Geometry check sheet. Reference: the model listing, model coordinates, mm. A direction names the side the tool comes from. Coordinates: 2 decimals unless noted, no trailing zeros. Loops run counter-clockwise (first coordinate to the right, second up) from the corner with the lowest first, then second, coordinate; pieces in that order, holes last. Notation, with made-up numbers: (-31.75, 29) -> (-0.75, 29) arc R20 cw to (-0.75, 56) -> close; hole circle Ø10 at (-30, 73.25). An arc over 180 degrees is marked (long way). Answer as a JSON object with one key per item and string values.
from build123d import *

# Parameters (mm, degrees)
SKETCH3_R          = 1.625
CUT_EXTRUDE1_DEPTH = 12
SKETCH4_R          = 2.1
CUT_EXTRUDE2_DEPTH = 10
CHAMFER1_SIZE      = 0.4
CHAMFER2_SIZE      = 0.4
CHAMFER3_SIZE      = 0.4
CHAMFER4_SIZE      = 0.3
CHAMFER5_SIZE      = 0.4


with BuildPart() as part:
    # Sketch2 → Revolve1 (revolve)
    with BuildSketch(Plane(origin=(0, 0, 0), x_dir=(1, 0, 0), z_dir=(0, 1, 0))):
        Polygon((0, 0), (0, 12), (-2.7, 12), (-2.7, 20.075), (-19.2, 20.075), (-19.2, 21.075), (-20.7, 21.075), (-20.7, 17.727837292), (-20.7, 14.575), (-20.7, 8.1), (-15.7, 8.1), (-15.7, 6), (-13.7, 6), (-13.7, 0), align=None)
    revolve(axis=Axis((0, 0, 0), (-1, 0, 0)))

    # Sketch3 → Cut-Extrude1 (cut)
    with BuildSketch(Plane.ZY.offset(20.7)):
        with Locations((0, 16)):
            Circle(SKETCH3_R)
        with Locations((13.856406461, 7.904729806)):
            Circle(SKETCH3_R)
        with Locations((13.773900052, -8.142905292)):
            Circle(SKETCH3_R)
        with Locations((-0.165012817, -16.095270194)):
            Circle(SKETCH3_R)
        with Locations((-14.021419278, -8)):
            Circle(SKETCH3_R)
        with Locations((-13.938912869, 8.047635097)):
            Circle(SKETCH3_R)
    extrude(amount=-CUT_EXTRUDE1_DEPTH, mode=Mode.SUBTRACT)

    # Sketch4 → Cut-Extrude2 (cut)
    with BuildSketch(Plane(origin=(-2.7, 0, 0), x_dir=(0, 0, -1), z_dir=(1, 0, 0))):
        with Locations((-8.125, 14.072912811)):
            Circle(SKETCH4_R)
        with Locations((8.125, 14.072912811)):
            Circle(SKETCH4_R)
        with Locations((16.25, 0)):
            Circle(SKETCH4_R)
        with Locations((8.125, -14.072912811)):
            Circle(SKETCH4_R)
        with Locations((-8.125, -14.072912811)):
            Circle(SKETCH4_R)
        with Locations((-16.25, 0)):
            Circle(SKETCH4_R)
    extrude(amount=-CUT_EXTRUDE2_DEPTH, mode=Mode.SUBTRACT)

    # Chamfer1
    chamfer1_edges = [part.edges().sort_by_distance(p)[0] for p in [
        (-2.7, 0, 20.075),
    ]]
    chamfer(chamfer1_edges, length=CHAMFER1_SIZE)

    # Chamfer2
    chamfer2_edges = [part.edges().sort_by_distance(p)[0] for p in [
        (-20.7, 0, 8.1),
    ]]
    chamfer(chamfer2_edges, length=CHAMFER2_SIZE)

    # Chamfer3
    chamfer3_edges = [part.edges().sort_by_distance(p)[0] for p in [
        (-20.7, 16, -1.625),
        (-20.7, 8.047635097, -15.563912869),
        (-20.7, -8, -15.646419278),
        (-20.7, -16.095270194, -1.790012817),
        (-20.7, -8.142905292, 12.148900052),
        (-20.7, 7.904729806, 12.231406461),
    ]]
    chamfer(chamfer3_edges, length=CHAMFER3_SIZE)

    # Chamfer4
    chamfer4_edges = [part.edges().sort_by_distance(p)[0] for p in [
        (-2.7, 0, 18.35),
        (-2.7, -14.072912811, 10.225),
        (-2.7, -14.072912811, -6.025),
        (-2.7, 0, -14.15),
        (-2.7, 14.072912811, -6.025),
        (-2.7, 14.072912811, 10.225),
    ]]
    chamfer(chamfer4_edges, length=CHAMFER4_SIZE)

    # Chamfer5
    chamfer5_edges = [part.edges().sort_by_distance(p)[0] for p in [
        (-20.7, 0, 21.075),
    ]]
    chamfer(chamfer5_edges, length=CHAMFER5_SIZE)


solid = part.part
1. Thickness scan on probe 1 along Z at (x, y) = (-12.5, -1); probe 2 along X at (y, z) = (-16.5, 10); probe 3 along Y at (x, z) = (-5, 0) (3 decimals). Record the ranges inside material, lowest first. Write a range as from..to.
Evaluation:
{"probe 1": "z = -20.05..-18.1, -14.4..14.4, 18.1..20.05", "probe 2": "x = -20.7..-2.7", "probe 3": "y = -20.075..20.075"}
2. Section check B-B, the plane x = -16.25. Record the boundary of the cut face in (y, z) (3 decimals).
Evaluation:
{"outline": "circle Ø40.15 at (0, 0); hole circle Ø3.25 at (-16.095, -0.165); hole circle Ø3.25 at (-8.143, 13.774); hole circle Ø3.25 at (-8, -14.021); hole circle Ø16.2 at (0, 0); hole circle Ø3.25 at (7.905, 13.856); hole circle Ø3.25 at (8.048, -13.939); hole circle Ø3.25 at (16, 0)"}
3. Mould release check, pull along Z, two halves, no side actions. Record for faces 1 (the face through (-19.758, 12.824, 16.724)), 2 (the face through (-15.7, 3, 5.4)): released by +Z, released by -Z, zero draft, split by the parting line, or undercut.
Evaluation:
{"face 1": "split by the parting line", "face 2": "undercut"}
4. Depth check by flat-ended pin: P1, Ø3, axis at x = -12, y = 2, coming from the -Z side; P2, Ø2, axis at x = -10, y = -16.5, coming from the +Z side; P3, Ø10, axis at x = -13.5, z = -16, coming from the +Y side. Enter the tip coordinate at first touch or a pass-through.
Evaluation:
{"P1": "stops at z = -20.07", "P2": "stops at z = 12.76", "P3": "stops at y = 16.79"}
5. Tool access check on faces 3 (the face through (-11.26, -6.03, -19.15)), 4 (the face through (-14.581, 6.916, 12.567)). Record the directions out of +Z, -Z, +X, -X, +Y, -Y that give a thin tool (end or side, any length) a straight path to the whole face; none if there is none.
Evaluation:
{"face 3": "+X", "face 4": "-X"}
6. Section check A-A, the plane x = -5.75. Record the boundary of the cut face in (y, z) (3 decimals).
Evaluation:
{"outline": "circle Ø40.15 at (0, 0); hole circle Ø4.2 at (-14.073, -8.125); hole circle Ø4.2 at (-14.073, 8.125); hole circle Ø4.2 at (0, -16.25); hole circle Ø4.2 at (0, 16.25); hole circle Ø4.2 at (14.073, -8.125); hole circle Ø4.2 at (14.073, 8.125)"}
